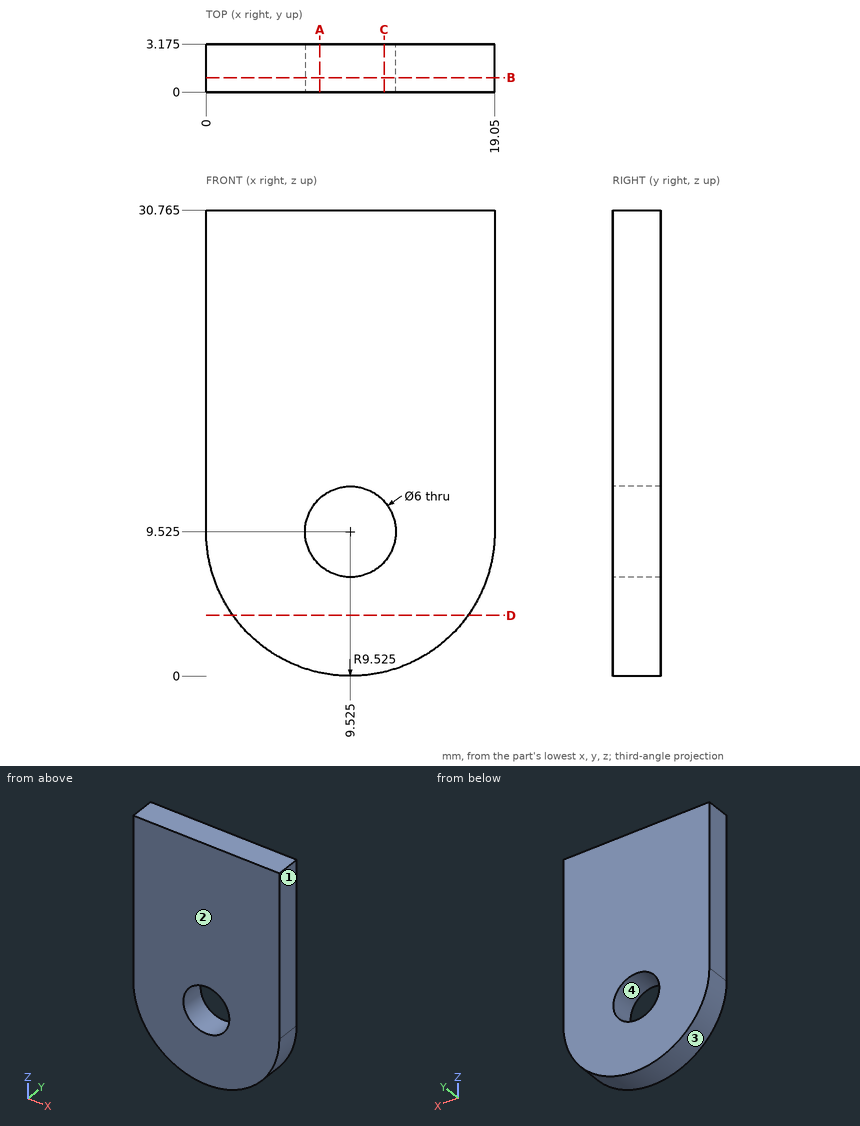
Answer from the drawing. Dimensions are ordinates in mm from the lowest x, y and z of the part. Give positions to 0.01 mm unless a question says otherwise; leave off trailing zeros. Write each loop counter-clockwise with the first axis right and the second up, starting at its lowest first coordinate (ties: lowest second). Pieces come first, ordered by that corner, then holes. Notation, with made-up numbers: (51.25, 64.25) - (95.25, 64.25) arc R17 ccw to (95.25, 68.25) - close; hole circle Ø10 at (79.25, -37.5). An arc over 180 degrees is marked (long way). One line per item, written item: value. Start each with the question number.
1. Find section A-A (x = 7.5). Write down the section's boundary in (y, z) (3 decimals).
2. For a pull along X with two mould halves and no side action, classify the marked faces 1, 2, 3 and 4 as +X half, -X half, draft (parallel to the pull), parting line (faces both ways), or undercut.
3. Consider probe 1 along Z at (x, y) = (10.5, 1.85) (3 decimals); probe 2 along Z at (x, y) = (8, 1.95) (3 decimals); probe 3 along Z at (x, y) = (1.75, 2.95) (3 decimals). Determine where each line is inside the solid, lowest interval first.
4. Find section C-C (x = 11.75). Write down the section's boundary in (y, z) (3 decimals), then the cut area to 3 significant figures.
5. Find section D-D (z = 4). Write down the section's boundary in (x, y) (3 decimals), then the cut area to 3 significant figures.
6. Find section B-B (y = 0.95). Write down the section's boundary in (x, z) (3 decimals), then the cut area to 3 significant figures.
Geometry results:
1. outline: (0, 0.218) - (3.175, 0.218) - (3.175, 7.312) - (0, 7.312) - close; (0, 11.738) - (3.175, 11.738) - (3.175, 30.765) - (0, 30.765) - close
2. face 1: +X half
2. face 2: draft
2. face 3: parting line
2. face 4: undercut
3. probe 1: 0.05 to 6.688, 12.362 to 30.765
3. probe 2: 0.123 to 6.942, 12.108 to 30.765
3. probe 3: 4.023 to 30.765
4. outline: (0, 0.264) - (3.175, 0.264) - (3.175, 7.513) - (0, 7.513) - close; (0, 11.537) - (3.175, 11.537) - (3.175, 30.765) - (0, 30.765) - close
4. area: 84.1 mm2
5. outline: (1.766, 0) - (17.284, 0) - (17.284, 3.175) - (1.766, 3.175) - close
5. area: 49.3 mm2
6. outline: (0, 9.525) arc R9.525 ccw to (19.05, 9.525) - (19.05, 30.765) - (0, 30.765) - close; hole circle Ø6 at (9.525, 9.525)
6. area: 519 mm2
